Read the model definition and answer for the solid it produces. Units are mm, in the model's axes. A direction names the side the tool comes from. Coordinates: 2 decimals unless noted, no trailing zeros. Write each loop counter-clockwise with the first axis right and the second up, starting at its lowest first coordinate (ties: lowest second). Pieces come first, ordered by that corner, then holes.
from build123d import *

# Parameters (mm, degrees)
F1_DEPTH  = 25.4
F2_W      = 24.5687300339
F2_H      = 2.9094554484
F3_DEPTH  = 25.4
F4_T      = -0.5
F5_R      = 3.0570054972
F5_R_2    = 3.0607
F6_R      = 3.181794186
F8_DEPTH  = 25.4
F9_R      = 12.1043942534
F10_DEPTH = 25.4


with BuildPart() as f1:
    # F0 (on Top) → F1 (new body)
    with BuildSketch(Plane.XY):
        with BuildLine():
            ThreePointArc((6.7371355302, 21.506121056), (14.414150376, 27.8790390368), (17.2925723513, 37.4323278666))
            ThreePointArc((17.2925723513, 37.4323278666), (-9.5532888298, 51.8464782426), (-6.7371355302, 21.506121056))
            ThreePointArc((-6.7371355302, 21.506121056), (0, 22.5366864917), (6.7371355302, 21.506121056))
        make_face()
        with BuildLine():
            ThreePointArc((15.3873619303, -16.4660660406), (0, -22.5366864917), (-15.3873619303, -16.4660660406))
            ThreePointArc((-15.3873619303, -16.4660660406), (-15.5425277668, -70.157586494), (30.9817265156, -43.3565191925))
            ThreePointArc((30.9817265156, -43.3565191925), (26.8010673015, -27.8139914256), (15.3873619303, -16.4660660406))
        make_face()
        with BuildLine():
            ThreePointArc((6.7371355302, 21.506121056), (0, 22.5366864917), (-6.7371355302, 21.506121056))
            ThreePointArc((-6.7371355302, 21.506121056), (0, 20.1397555152), (6.7371355302, 21.506121056))
        make_face()
        with BuildLine():
            ThreePointArc((6.7371355302, 21.506121056), (0, 20.1397555152), (-6.7371355302, 21.506121056))
            ThreePointArc((-6.7371355302, 21.506121056), (-21.9737364868, 5.0057110217), (-15.3873619303, -16.4660660406))
            ThreePointArc((-15.3873619303, -16.4660660406), (0, -12.3747926769), (15.3873619303, -16.4660660406))
            ThreePointArc((15.3873619303, -16.4660660406), (20.6722324603, -8.9755803787), (22.5366864917, 0))
            ThreePointArc((22.5366864917, 0), (18.1622541184, 13.3429668127), (6.7371355302, 21.506121056))
        make_face()
        with BuildLine():
            ThreePointArc((15.3873619303, -16.4660660406), (0, -12.3747926769), (-15.3873619303, -16.4660660406))
            ThreePointArc((-15.3873619303, -16.4660660406), (0, -22.5366864917), (15.3873619303, -16.4660660406))
        make_face()
    extrude(amount=F1_DEPTH)

    # F2 (on Top) → F3 (cut)
    with BuildSketch(Plane.XY):
        with Locations((4.657e-07, 54.3079804629)):
            Rectangle(F2_W, F2_H)
    extrude(amount=F3_DEPTH, mode=Mode.SUBTRACT)

    # F4 (hollow: no face is removed)
    offset(amount=F4_T, kind=Kind.INTERSECTION, mode=Mode.SUBTRACT)

    # F5 (on face) + F6 (on face) + F7 (on face) → F8 (cut)
    with BuildSketch(Plane.XY.offset(25.4)):
        with Locations((0, 13.8647966087)):
            Circle(F5_R)
        with Locations((0, 1.6805409687)):
            Circle(F5_R_2)
        with Locations((0, -11.7677608505)):
            Circle(F5_R_2)
    with BuildSketch(Plane.XY.offset(25.4)):
        with Locations((-4.9822856672, 42.3047989607)):
            Circle(F6_R)
        with Locations((4.9822856672, 42.3047989607)):
            Circle(F6_R)
    with BuildSketch(Plane.XY.offset(25.4)):
        with BuildLine():
            ThreePointArc((7.2696800344, 31.6944643855), (-0.4129284645, 30.2212155736), (-8.011739701, 32.0789031684))
            ThreePointArc((-8.011739701, 32.0789031684), (-0.4918764169, 27.0830389619), (7.2696800344, 31.6944643855))
        make_face()
    extrude(amount=-F8_DEPTH, mode=Mode.SUBTRACT)

    # F9 (on face) → F10 (cut)
    with BuildSketch(Plane(origin=(0, 52.8532527387, 0), x_dir=(-1, 0, 0), z_dir=(0, 1, 0))):
        with Locations((0, 12.44416181)):
            Circle(F9_R)
    extrude(amount=-F10_DEPTH, mode=Mode.SUBTRACT)


solid = f1.part
Item 1: Given pin 1 (4 mm diameter, centred on y = -34.5, z = 5, fed in from -X); pin 2 (7.5 mm diameter, centred on x = -4.98, y = 42.3, fed in from +Z); pin 3 (10 mm diameter, centred on y = -27.5, z = 11.5, fed in from -X); pin 4 (2 mm diameter, centred on y = -5, z = 14.5, fed in from -X), each flat-ended and moving along its own axis, determine where each tip first touches the part or whether it passes through.
Item 2: Determine the mould class of faces 1 (the cylindrical face through (-17.29, 37.11, 12.52)), 2 (the flat face through (-0.11, 52.853, 0.16)), 3 (the cylindrical face through (-5.4, 45.46, 0.25)) for opening direction Y: +Y half, -Y half, draft (parallel to the pull), parting line (faces both ways), or undercut.
Item 3: The part is cut by section A-A (y = 12). Give the vertices of the cut face in (x, z).
Item 4: The part is cut by section B-B (x = -24.5). Give the vertices of the cut face in (y, z).
Item 5: The part is cut by section C-C (y = -57.5). Give the vertices of the cut face in (x, z) (3 decimals).
Item 6: The part is cut by section D-D (z = 5.25). Give the vertices of the cut face in (x, y), and give its area (3 significant figures).
Item 7: Find the intervals of material crossed by probe 1 along Y at (x, z) = (0, 25.35); probe 2 along Y at (x, z) = (7.5, 8); probe 3 along Y at (x, z) = (-8, 13.25), in increasing order.
Item 8: For faces 4 (the cylindrical face through (-21.305, 5.632, 12.529)), 5 (the cylindrical face through (2.92, -10.85, 0.25)), 6 (the cylindrical face through (-0.53, 45.78, 0.35)), determine the directions among +Z, -Z, +X, -X, +Y, -Y from which every point of the face is accessible in a straight line to the end or side of a thin tool.
Answer:
1. pin 1: stops at x = -30.21
1. pin 2: stops at z = 25.4
1. pin 3: stops at x = -29.02
1. pin 4: stops at x = -22.18
2. face 1: undercut
2. face 2: +Y half
2. face 3: undercut
3. outline: (-19.08, 0) - (-2.42, 0) - (-2.42, 0.5) - (-18.48, 0.5) - (-18.48, 24.9) - (-2.42, 24.9) - (-2.42, 25.4) - (-19.08, 25.4) - close; (2.42, 0) - (19.08, 0) - (19.08, 25.4) - (2.42, 25.4) - (2.42, 24.9) - (18.48, 24.9) - (18.48, 0.5) - (2.42, 0.5) - close
4. outline: (-62.32, 0) - (-24.39, 0) - (-24.39, 25.4) - (-62.32, 25.4) - close; hole (-61.49, 0.5) - (-25.22, 0.5) - (-25.22, 24.9) - (-61.49, 24.9) - close
5. outline: (-27.565, 0) - (27.565, 0) - (27.565, 25.4) - (-27.565, 25.4) - close; hole (-27.002, 0.5) - (27.002, 0.5) - (27.002, 24.9) - (-27.002, 24.9) - close
6. outline: (-15.39, -16.47) arc R30.98 ccw (long way) to (15.39, -16.47) arc R22.54 ccw to (6.74, 21.51) arc R17.29 ccw to (9.73, 51.72) - (9.73, 51.12) arc R16.79 cw to (5.11, 21.44) arc R22.04 cw to (14.54, -16.56) arc R30.48 cw (long way) to (-14.54, -16.56) arc R22.04 cw to (-5.11, 21.44) arc R16.79 cw to (-9.73, 51.12) - (-9.73, 51.72) arc R17.29 ccw to (-6.74, 21.51) arc R22.54 ccw to start
6. area: 166 mm2
7. probe 1: y = -74.34 to -14.83, -8.71 to -1.38, 4.74 to 10.81, 16.92 to 27.08, 30.22 to 52.85
7. probe 2: y = -73.42 to -72.9, 20.72 to 21.25, 21.85 to 22.41
7. probe 3: y = -73.29 to -72.77, 20.53 to 21.07, 22.1 to 22.67
8. face 4: none
8. face 5: +Z, -Z
8. face 6: +Y
